For this review, use the dimensioned drawing (mm, ordinates from the lowest corner) and the shaded views. A direction names the side the tool comes from. Give positions to 0.01 mm unless a question says otherwise; leave off trailing zeros. Write each loop counter-clockwise with the first axis right and the second up, starting at its lowest first coordinate (ties: lowest second). Pieces come first, ordered by that corner, then holes.
1) We need section B-B on y = 2.5. Give the boundary of the cut face in (x, z).
2) We need section D-D on y = 7. Give the boundary of the cut face in (x, z), and give its area (3 significant figures).
3) For P1, Ø1.5, axis at x = 5, y = 2, coming from the +Z side; P2, Ø4, axis at x = 18.5, y = 2, coming from the -Z side; P3, Ø4, axis at y = 3, z = 9, coming from the -X side, all flat-tipped, find the tip position at first contact; note any pin that passes through.
4) Machinability: for the marked faces 4, 5 and 6, which of the approach directions +Z, -Z, +X, -X, +Y, -Y give a long, thin tool a straight path to every point of the face, cutting with its end or side? Answer none if there is none.
5) Draft analysis for pull direction X (two halves, no side actions). For the marked faces 1, 2 and 3, state which applies: pulls with the +X half, pulls with the -X half, needs draft (parallel to the pull), parting line crosses it, or undercut.
6) We need section A-A on x = 2.5. Give the boundary of the cut face in (y, z).
7) We need section C-C on z = 3.5. Give the boundary of the cut face in (x, y), and give its area (3 significant figures).
8) Wall thickness on line 1 along Y through (x, z) = (2.5, 2.65); line 2 along X through (y, z) = (11.5, 8.75); line 3 along Z through (x, y) = (8, 6.75): over which ranges is each line inside the solid? List them lowest first.
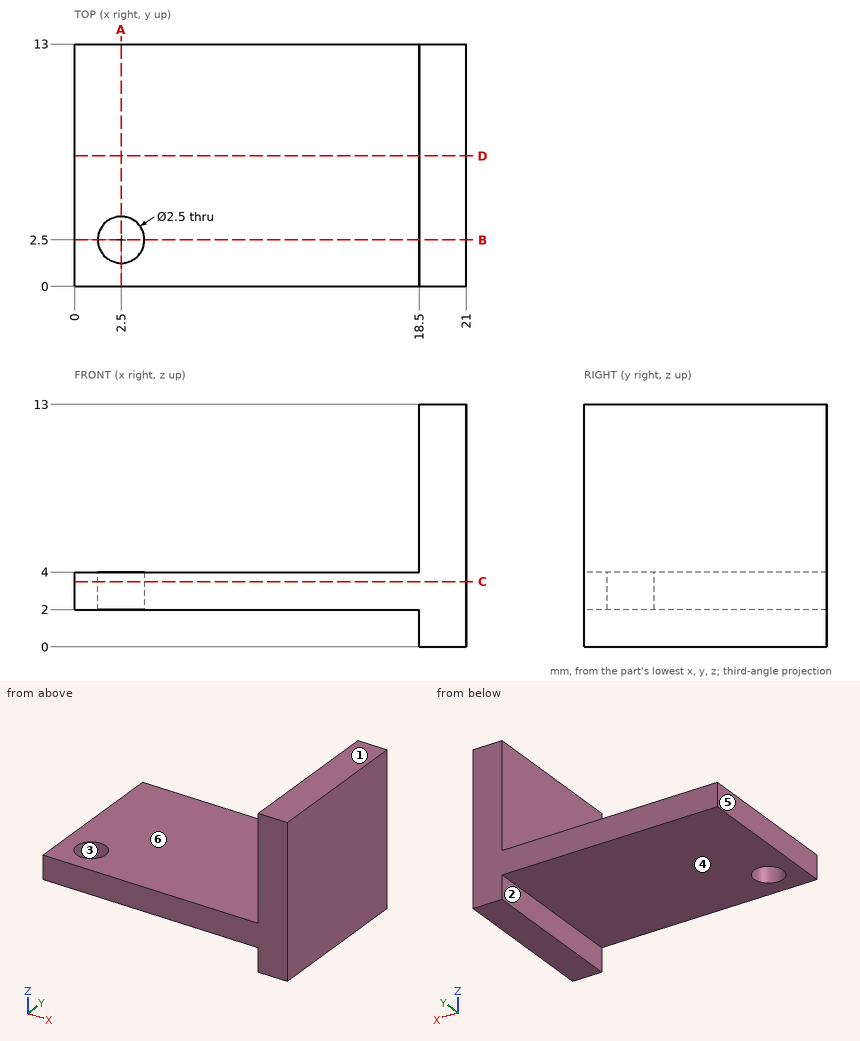
Results list:
1. outline: (0, 2) - (1.25, 2) - (1.25, 4) - (0, 4) - close; (3.75, 2) - (18.5, 2) - (18.5, 0) - (21, 0) - (21, 13) - (18.5, 13) - (18.5, 4) - (3.75, 4) - close
2. outline: (0, 2) - (18.5, 2) - (18.5, 0) - (21, 0) - (21, 13) - (18.5, 13) - (18.5, 4) - (0, 4) - close
2. area: 69.5 mm2
3. P1: stops at z = 4
3. P2: stops at z = 0
3. P3: stops at x = 18.5
4. face 4: -Z, -X, +Y, -Y
4. face 5: +Z, -Z, -X, +Y, -Y
4. face 6: +Z, -X, +Y, -Y
5. face 1: needs draft
5. face 2: pulls with the -X half
5. face 3: undercut
6. outline: (0, 2) - (1.25, 2) - (1.25, 4) - (0, 4) - close; (3.75, 2) - (13, 2) - (13, 4) - (3.75, 4) - close
7. outline: (0, 0) - (21, 0) - (21, 13) - (0, 13) - close; hole circle Ø2.5 at (2.5, 2.5)
7. area: 268 mm2
8. line 1: y = 0 to 1.25, 3.75 to 13
8. line 2: x = 18.5 to 21
8. line 3: z = 2 to 4
